Verification items for the finished model (mm, model axes). A direction names the side the tool comes from. Round coordinates to 2 decimals unless told otherwise and drop trailing zeros. Loops run counter-clockwise (first coordinate to the right, second up) from the corner with the lowest first, then second, coordinate; pieces in that order, holes last. Notation, with made-up numbers: (-17, -5.5) - (8, -5.5) arc R20 ccw to (8, 3.5) - close; hole circle Ø7 at (9.5, -35). An arc over 180 degrees is marked (long way). Use CSV: the item, a comma, the result in double quotes.
```python
from build123d import *

# Parameters (mm, degrees)
SKETCH_W     = 36
SKETCH_H     = 26
SKETCH_R     = 1.5
SKETCH_R_2   = 0.75
PAD_DEPTH    = 1.5
PAD001_DEPTH = 1.5
SKETCH002_W  = 1
SKETCH002_H  = 1
PAD002_DEPTH = 3.5
CHAMFER_SIZE = 0.25


with BuildPart() as part:
    # Sketch → Pad (new body)
    with BuildSketch(Plane.XY):
        Rectangle(SKETCH_W, SKETCH_H)
        with Locations((-14.5, 9.5)):
            Circle(SKETCH_R, mode=Mode.SUBTRACT)
        with Locations((14.5, 9.5)):
            Circle(SKETCH_R, mode=Mode.SUBTRACT)
        with Locations((14.5, -9.5)):
            Circle(SKETCH_R, mode=Mode.SUBTRACT)
        with Locations((-14.5, -9.5)):
            Circle(SKETCH_R, mode=Mode.SUBTRACT)
        with Locations((-16.5, 3.81)):
            Circle(SKETCH_R_2, mode=Mode.SUBTRACT)
        with Locations((-16.5, 1.27)):
            Circle(SKETCH_R_2, mode=Mode.SUBTRACT)
        with Locations((-16.5, -1.27)):
            Circle(SKETCH_R_2, mode=Mode.SUBTRACT)
        with Locations((-16.5, -3.81)):
            Circle(SKETCH_R_2, mode=Mode.SUBTRACT)
    extrude(amount=PAD_DEPTH)

    # Sketch001 (on Face13 of Pad) → Pad001 (join)
    with BuildSketch(Plane(origin=(0, 0, 0), x_dir=(1, 0, 0), z_dir=(0, 0, -1))):
        Polygon((-17.77, 4.726447), (-17.77, 2.893553), (-17.416447, 2.54), (-15.583553, 2.54), (-15.23, 2.893553), (-15.23, 4.726447), (-15.583553, 5.08), (-17.416447, 5.08), align=None)
        Polygon((-17.77, 2.186447), (-17.77, 0.353553), (-17.416447, 0), (-15.583553, 0), (-15.23, 0.353553), (-15.23, 2.186447), (-15.583553, 2.54), (-17.416447, 2.54), align=None)
        Polygon((-17.77, -0.353553), (-17.77, -2.186447), (-17.416447, -2.54), (-15.583553, -2.54), (-15.23, -2.186447), (-15.23, -0.353553), (-15.583553, 0), (-17.416447, 0), align=None)
        Polygon((-17.77, -2.893553), (-17.77, -4.726447), (-17.416447, -5.08), (-15.583553, -5.08), (-15.23, -4.726447), (-15.23, -2.893553), (-15.583553, -2.54), (-17.416447, -2.54), align=None)
    extrude(amount=PAD001_DEPTH)

    # Sketch002 (on Face41 of Pad001) → Pad002 (join, symmetric)
    with BuildSketch(Plane(origin=(0, 0, -1.5), x_dir=(1, 0, 0), z_dir=(0, 0, -1))):
        with Locations((-16.5, 3.81)):
            Rectangle(SKETCH002_W, SKETCH002_H)
        with Locations((-16.5, 1.27)):
            Rectangle(SKETCH002_W, SKETCH002_H)
        with Locations((-16.5, -1.27)):
            Rectangle(SKETCH002_W, SKETCH002_H)
        with Locations((-16.5, -3.81)):
            Rectangle(SKETCH002_W, SKETCH002_H)
    extrude(amount=PAD002_DEPTH, both=True)

    # Chamfer
    chamfer_edges = [part.edges().sort_by_distance(p)[0] for p in [
        (-16, 1.27, 2),
        (-16, 3.81, 2),
        (-16.5, 4.31, 2),
        (-17, 3.81, 2),
        (-16.5, 3.31, 2),
        (-16.5, 1.77, 2),
        (-17, 1.27, 2),
        (-16.5, 0.77, 2),
        (-17, -1.27, 2),
        (-16.5, -0.77, 2),
        (-16, -1.27, 2),
        (-16.5, -1.77, 2),
        (-16.5, -3.31, 2),
        (-17, -3.81, 2),
        (-16.5, -4.31, 2),
        (-16, -3.81, 2),
        (-16, -1.27, -5),
        (-16, -3.81, -5),
        (-16.5, -4.31, -5),
        (-17, -3.81, -5),
        (-16.5, -3.31, -5),
        (-16.5, -1.77, -5),
        (-17, -1.27, -5),
        (-16.5, -0.77, -5),
        (-16.5, 0.77, -5),
        (-16, 1.27, -5),
        (-16.5, 1.77, -5),
        (-17, 1.27, -5),
        (-16.5, 3.31, -5),
        (-16, 3.81, -5),
        (-16.5, 4.31, -5),
        (-17, 3.81, -5),
    ]]
    chamfer(chamfer_edges, length=CHAMFER_SIZE)


solid = part.part
```
1) Thickness scan on probe 1 along Y at (x, z) = (14.5, 1.1); probe 2 along Y at (x, z) = (-13.5, 0.5); probe 3 along Z at (x, y) = (13, 10.75). Record the ranges inside material, lowest first. Write a range as [from, to].
Returned:
probe 1,"y = [-13, -11], [-8, 8], [11, 13]"
probe 2,"y = [-13, -10.62], [-8.38, 8.38], [10.62, 13]"
probe 3,"z = [0, 1.5]"
2) Mould release check, pull along Y, two halves, no side actions. Record for faces 4 (the face through (-15.23, -1, -1)), 5 (the face through (-16, -5.08, -1)), 6 (the face through (-16.5, 4.31, 0.9)), 7 (the face through (-16.5, 3.31, -3.1)): +Y half, -Y half, draft (parallel to the pull), parting line (faces both ways), or undercut.
Returned:
face 4,"draft"
face 5,"-Y half"
face 6,"undercut"
face 7,"undercut"
3) Cross-section at B-B, the plane z = -4. Record the cut outline in (x, y), then the cut area to 3 significant figures.
Returned:
outline,"(-17, -4.31) - (-16, -4.31) - (-16, -3.31) - (-17, -3.31) - close; (-17, -1.77) - (-16, -1.77) - (-16, -0.77) - (-17, -0.77) - close; (-17, 0.77) - (-16, 0.77) - (-16, 1.77) - (-17, 1.77) - close; (-17, 3.31) - (-16, 3.31) - (-16, 4.31) - (-17, 4.31) - close"
area,"4.00 mm²"
4) Cross-section at C-C, the plane y = -9.5. Record the cut outline in (x, z).
Returned:
outline,"(-18, 0) - (-16, 0) - (-16, 1.5) - (-18, 1.5) - close; (-13, 0) - (13, 0) - (13, 1.5) - (-13, 1.5) - close; (16, 0) - (18, 0) - (18, 1.5) - (16, 1.5) - close"
5) Cross-section at A-A, the plane x = 14.5. Record the cut outline in (y, z).
Returned:
outline,"(-13, 0) - (-11, 0) - (-11, 1.5) - (-13, 1.5) - close; (-8, 0) - (8, 0) - (8, 1.5) - (-8, 1.5) - close; (11, 0) - (13, 0) - (13, 1.5) - (11, 1.5) - close"
6) Access from +Z, -Z, +X, -X, +Y, -Y to the whole of each face (thin tool, end or side, straight path). Record for faces 1 (the face through (-16.5, 3.31, 0.9)), 2 (the face through (-15.7, -10.4, 0.7)), 3 (the face through (-16.5, 0.77, -3.1)).
Returned:
face 1,"+Z"
face 2,"+Z, -Z"
face 3,"-Z, +X, -X"
7) Cross-section at D-D, the plane y = -5.5. Record the cut outline in (x, z), then the cut area to 3 significant figures.
Returned:
outline,"(-18, 0) - (18, 0) - (18, 1.5) - (-18, 1.5) - close"
area,"54.0 mm²"
8) Gauge pin test, flat ends, axial feed: pin 1 Ø0.8 at (y, z) = (3.5, -3.5) entering from -X; pin 2 Ø4 at (x, y) = (14.5, 9.5) entering from +Z; pin 3 Ø1 at (x, y) = (7.5, -2) entering from -Z. Record the tip position at first contact, or that the pin passes through.
Returned:
pin 1,"stops at x = -17"
pin 2,"stops at z = 1.5"
pin 3,"stops at z = 0"
